```python
from build123d import *

# Parameters (mm, degrees)
BOSS_EXTRUDE1_DEPTH = 150
CUT_EXTRUDE1_DEPTH  = 368.015632897
BOSS_EXTRUDE3_DEPTH = 5
BOSS_EXTRUDE4_START = 70
BOSS_EXTRUDE4_DEPTH = 20
SKETCH6_R           = 30
SKETCH6_R_2         = 20
BOSS_EXTRUDE5_DEPTH = 90


with BuildPart() as part:
    # Sketch1 → Boss-Extrude1 (new body, symmetric)
    with BuildSketch(Plane.XY):
        with BuildLine():
            Line((0, 0), (-269.007095808, 0))
            ThreePointArc((-269.007095808, 0), (-385.585141332, 59.468589851), (-405.875242761, 188.756120808))
            Line((-405.875242761, 188.756120808), (-362.32962564, 321.922441203))
            Line((-362.32962564, 321.922441203), (-224.01265789, 321))
            Line((-224.01265789, 321), (-223.905955644, 336.999644203))
            Line((-223.905955644, 336.999644203), (-373.905955644, 338))
            Line((-373.905955644, 338), (-421.082814644, 193.72902312))
            ThreePointArc((-421.082814644, 193.72902312), (-398.538257501, 50.076210945), (-269.007095808, -16))
            Line((-269.007095808, -16), (13, -16))
            Line((13, -16), (0, 0))
        make_face()
    extrude(amount=BOSS_EXTRUDE1_DEPTH, both=True)

    # Sketch2 → Cut-Extrude1 (cut, through all)
    with BuildSketch(Plane(origin=(1.559593234, 1.046677898, 0), x_dir=(0, 0, -1), z_dir=(0.83033878, 0.557258925, 0))):
        Polygon((-150, -20.529786514), (-140, 489.016938742), (-150, 489.016938742), align=None)
        Polygon((140, 489.016938742), (150, 489.016938742), (150, -20.529786514), align=None)
    extrude(amount=-CUT_EXTRUDE1_DEPTH, mode=Mode.SUBTRACT)

    # Sketch4 → Boss-Extrude3 (add)
    with BuildSketch(Plane(origin=(-1.635418654, 2.436841241, 149.539501663), x_dir=(0.999940218, 0.000134312, 0.010933523), z_dir=(-0.01093426, 0.016292498, 0.99980748))):
        with BuildLine():
            Line((14.637102301, -18.441255084), (-267.38685506, -18.403370819))
            add(Edge.make_bspline(
                [(-419.48086469, 191.373926331), (-488.057520629, -18.373728139), (-267.38685506, -18.403370819)],
                knots=[0.663674022, 0.663674022, 0.663674022, 2.550511677, 2.550511677, 2.550511677], degree=2, weights=[1, 0.587023682, 1]))
            Line((-419.48086469, 191.373926331), (-372.30751216, 335.657719572))
            Line((-372.30751216, 335.657719572), (-222.298499603, 334.637080266))
            Line((-222.298499603, 334.637080266), (14.637102301, -18.441255084))
        make_face()
    boss_extrude3 = extrude(amount=BOSS_EXTRUDE3_DEPTH)

    # Sketch5 → Boss-Extrude4 (add)
    with BuildSketch(Plane.XY.offset(BOSS_EXTRUDE4_START)):
        with BuildLine():
            Line((-373.905955644, 338), (-223.905955644, 336.999644203))
            Line((-223.905955644, 336.999644203), (-249.503039478, 448.668975164))
            ThreePointArc((-249.503039478, 448.668975164), (-297.905622093, 487.496486507), (-346.8217607, 449.317997476))
            Line((-346.8217607, 449.317997476), (-373.905955644, 338))
        make_face()
        with BuildLine():
            Line((-421.082814644, 193.72902312), (-515.85308915, 263.184838763))
            ThreePointArc((-515.85308915, 263.184838763), (-530.093343715, 308.281281099), (-491.377505751, 335.439297452))
            Line((-491.377505751, 335.439297452), (-373.905955644, 333))
            Line((-373.905955644, 333), (-421.082814644, 193.72902312))
        make_face()
    boss_extrude4 = extrude(amount=BOSS_EXTRUDE4_DEPTH)

    # Mirror4: Boss-Extrude3, Boss-Extrude4 across plane
    add(boss_extrude3.mirror(Plane.XY))
    add(boss_extrude4.mirror(Plane.XY))

    # Sketch6 → Boss-Extrude5 (add, symmetric)
    with BuildSketch(Plane.XY):
        with Locations((-298.23906661, 437.497598372)):
            Circle(SKETCH6_R)
        with Locations((-492.207926981, 295.447918374)):
            Circle(SKETCH6_R_2)
    extrude(amount=BOSS_EXTRUDE5_DEPTH, both=True)


solid = part.part
```
CAD build for the part. Positions are in the model's coordinates, mm. A direction names the side the tool comes from. Give positions to 0.01 mm unless a question says otherwise; leave off trailing zeros. Write each loop counter-clockwise with the first axis right and the second up, starting at its lowest first coordinate (ties: lowest second). Pieces come first, ordered by that corner, then holes. Notation, with made-up numbers: (-5, 6) -> (18, 6) arc R10 ccw to (18, 12) -> close; hole circle Ø8 at (56.25, 60.5). An arc over 180 degrees is marked (long way). Write each question's results on one line, items separated by ' | '.
1. Cut at A-A, the plane z = -78. Write the cut outline in (x, y), then the cut area to 3 significant figures.
Geometry check:
outline: (-515.85, 263.18) -> (-421.08, 193.73) arc R160 ccw to (-269.01, -16) -> (13, -16) -> (0, 0) -> (-269.01, 0) arc R144 cw to (-405.88, 188.76) -> (-362.33, 321.92) -> (-224.01, 321) -> (-223.91, 337) -> (-249.5, 448.67) arc R50 ccw to (-346.82, 449.32) -> (-373.91, 338) -> (-375.53, 333.03) -> (-491.38, 335.44) arc R40 ccw to start | area: 44,200 mm²
2. Cut at C-C, the plane z = -30.5. Write the cut outline in (x, y).
Geometry check:
outline: circle Ø40 at (-492.21, 295.45); (-421.08, 193.73) arc R160 ccw to (-269.01, -16) -> (13, -16) -> (0, 0) -> (-269.01, 0) arc R144 cw to (-405.88, 188.76) -> (-362.33, 321.92) -> (-224.01, 321) -> (-223.91, 337) -> (-373.91, 338) -> close; circle Ø60 at (-298.24, 437.5)
3. Two-plate mould, pull along X, no slides. Class faces 6 (the flat face through (-397.164, 266.874, 1.986)), 7 (the flat face through (-360.174, 394.438, 79.86)), 8 (the flat face through (-300, 397, -90)): pulls with the +X half, pulls with the -X half, needs draft (parallel to the pull), parting line crosses it, or undercut.
Geometry check:
face 6: undercut | face 7: pulls with the -X half | face 8: needs draft
4. Cut at D-D, the plane x = -100. Write the cut outline in (y, z).
Geometry check:
outline: (-16, -148.76) -> (-15.92, -153.76) -> (152.37, -151.02) -> (152.37, -146.02) -> (0, -148.5) -> (0, 148.5) -> (152.37, 146.02) -> (152.37, 151.02) -> (-15.92, 153.76) -> (-16, 148.76) -> close
5. Which spindle directions (+Z, -Z, +X, -X, +Y, -Y) get a long thin tool onto all of the face, cutting with end or side? Do faces 1 (the flat face through (6.59, -8.11, 2.1)), 2 (the flat face through (-300, 397, 90)), 3 (the flat face through (-130, -16, 2)), 4 (the cylindrical face through (-296.97, 487.48, -79.86)), 5 (the flat face through (-300, 397, -70)). Say none if no direction does.
Geometry check:
face 1: +X, +Y | face 2: +Z, +X, -X, +Y | face 3: +Z, -Z, +X, -X, -Y | face 4: +Z, -Z, +Y | face 5: none
6. Cut at B-B, the plane y = 397. Write the cut outline in (x, z), then the cut area to 3 significant figures.
Geometry check:
outline: (-359.55, -90) -> (-237.66, -90) -> (-237.66, -70) -> (-359.55, -70) -> close; (-359.55, 70) -> (-237.66, 70) -> (-237.66, 90) -> (-359.55, 90) -> close | area: 4,880 mm²
7. Drop flat-ended pins along their axis: P1, Ø4, axis at y = 434.5, z = -22.5, coming from the -X side; P2, Ø10, axis at x = -473, y = 285, coming from the +Z side; P3, Ø12, axis at y = 215, z = 10.5, coming from the +X side. Give the stop position or say it passes through.
Geometry check:
P1: x = -328.22 | P2: z = 90 | P3: x = -395.33
8. Wall check: probe 1 along Z at (x, y) = (-488, 248); probe 2 along Y at (x, z) = (-240, 67); probe 3 along Z at (x, y) = (-159.5, 63). Give the ranges that are in metal, low to high. Write a range as [from, to].
Geometry check:
probe 1: [-90, -70], [70, 90] | probe 2: [-16, 0], [321.11, 337.11] | probe 3: [-151.83, -146.83], [146.83, 151.83]
